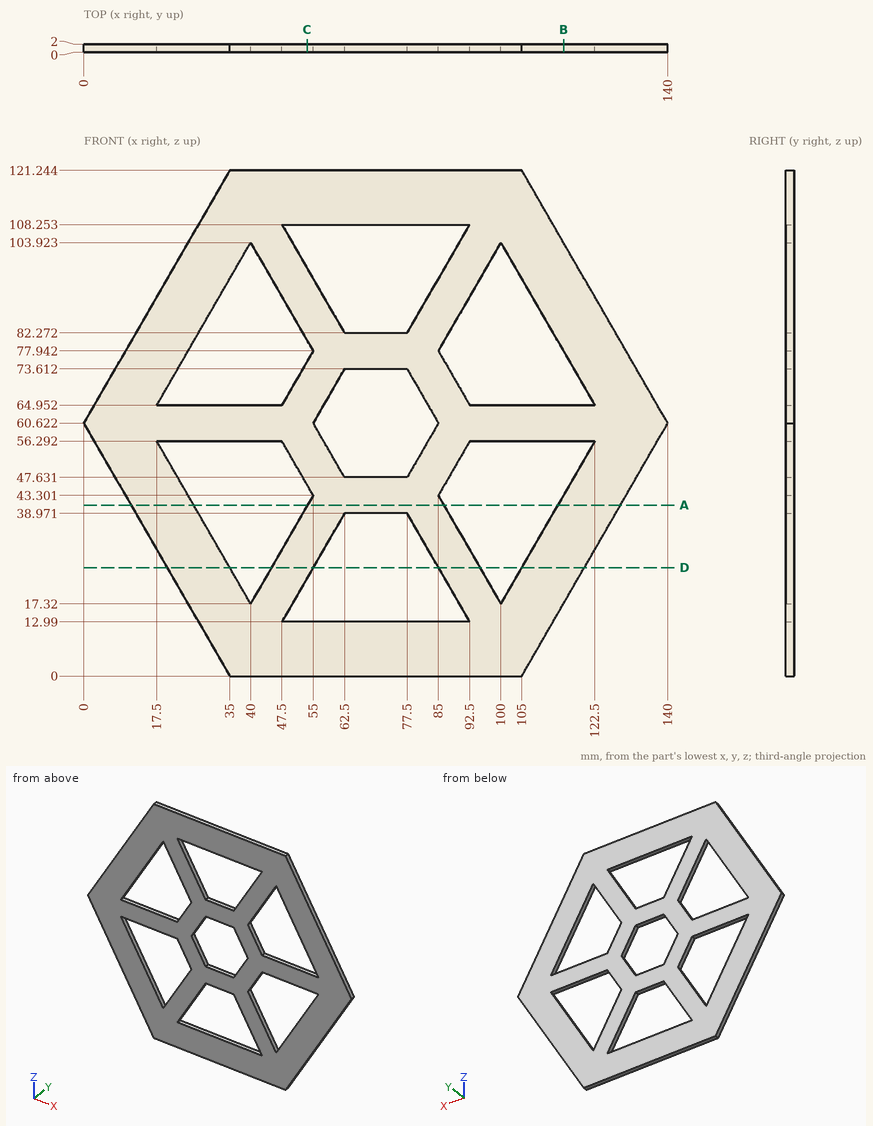
Can you work these out from the drawing? Everything is in mm from the part's minimum corner. Give positions to 0.01 mm unless a question says otherwise; leave off trailing zeros. Order: outer loops, then holes, each group sorted by start corner. A loop starts at its lowest first (then second) coordinate and runs counter-clockwise, first axis right, second up. Notation, with made-up numbers: M 25,80.25 L 65,80.25 A22 ccw 65,101.25 Z; hole C -38,84 d9. An arc over 180 degrees is marked long. Use a Markdown table: item, result. Add a question column.
1. Suppose I cut it at D-D (z = 26). List the corners of the cut face in (x, y) for me.
2. Suppose I cut it at C-C (x = 53.5). List the corners of the cut face in (y, z) for me (1 decimal), and give its area (3 significant figures).
3. Suppose I cut it at B-B (x = 115). List the corners of the cut face in (y, z) for me.
4. I need wall thicknesses on probe 1 along Z at (x, y) = (76, 1.1); probe 2 along X at (y, z) = (1.3, 89) (1 decimal); probe 3 along X at (y, z) = (1.5, 73.5) (1 decimal). Which ranges of each line are inside material? Lowest first, please. Write a range as from..to.
5. For pin 1 Ø0.6 at (x, y) = (34, 0.5) entering from -Z (1 decimal), with a flat end and sliding along its axis, tell me the tip position at first contact or that it passes through.
6. Suppose I cut it at A-A (z = 41). List the corners of the cut face in (x, y) for me.
Results list:
| question | item | result |
|---|---|---|
| 1 | outline | M 19.99,0 L 34.99,0 L 34.99,2 L 19.99,2 Z; M 45.01,0 L 55.01,0 L 55.01,2 L 45.01,2 Z; M 84.99,0 L 94.99,0 L 94.99,2 L 84.99,2 Z; M 105.01,0 L 120.01,0 L 120.01,2 L 105.01,2 Z |
| 2 | outline | M 0,0 L 2,0 L 2,13 L 0,13 Z; M 0,23.4 L 2,23.4 L 2,40.7 L 0,40.7 Z; M 0,45.9 L 2,45.9 L 2,75.3 L 0,75.3 Z; M 0,80.5 L 2,80.5 L 2,97.9 L 0,97.9 Z; M 0,108.3 L 2,108.3 L 2,121.2 L 0,121.2 Z |
| 2 | area | 180 mm² |
| 3 | outline | M 0,17.32 L 2,17.32 L 2,43.3 L 0,43.3 Z; M 0,56.29 L 2,56.29 L 2,64.95 L 0,64.95 Z; M 0,77.94 L 2,77.94 L 2,103.92 L 0,103.92 Z |
| 4 | probe 1 | z = 0..12.99, 38.97..47.63, 73.61..82.27, 108.25..121.24 |
| 4 | probe 2 | x = 16.4..31.4, 48.6..58.6, 81.4..91.4, 108.6..123.6 |
| 4 | probe 3 | x = 7.4..22.4, 52.4..62.4, 77.6..87.6, 117.6..132.6 |
| 5 | pin 1 | stops at z = 1.2 |
| 6 | outline | M 11.33,0 L 26.33,0 L 26.33,2 L 11.33,2 Z; M 53.67,0 L 86.33,0 L 86.33,2 L 53.67,2 Z; M 113.67,0 L 128.67,0 L 128.67,2 L 113.67,2 Z |
